Answer from the drawing. Dimensions are ordinates in mm from the lowest x, y and z of the part. Round coordinates to 2 decimals unless told otherwise and drop trailing zeros. Write each loop counter-clockwise with the first axis right and the second up, starting at its lowest first coordinate (ties: lowest second). Pieces come first, ordered by that corner, then holes. Notation, with made-up numbers: (-38, 32.5) -> (-1, 32.5) arc R21 cw to (-1, 56.5) -> close; hole circle Ø1 at (-27, 5). An arc over 180 degrees is marked (long way). Answer as a JSON object with one key per item and string values. Group by question number.
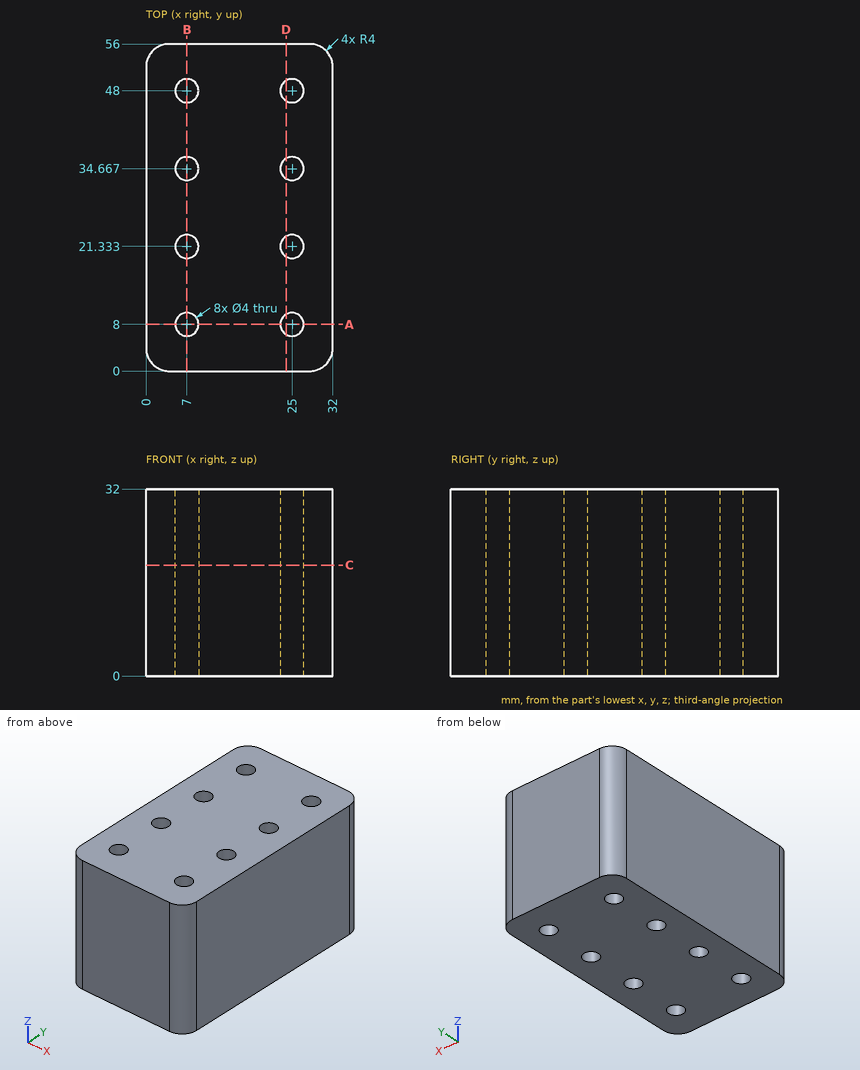
1) A cutting plane is placed at D-D on x = 24. Determine the outline of the cut face in (y, z) (1 decimal), plus the area to 3 significant figures.
2) Straight lines are drawn through the part: L1, parallel to Y at x = 25, z = 9.5; L2, parallel to X at y = 34.5, z = 14.5; L3, parallel to Y at x = 8.5, z = 15 (1 decimal). For each, find the intervals that lie inside material, in ascending order.
3) This flat-tipped pin is pushed along its axis until it touches: P1, Ø10, axis at x = 4.5, z = 7, coming from the -Y side. Where does it stop, or does it pass through?
4) A cutting plane is placed at A-A on y = 8. Determine the outline of the cut face in (x, z).
5) A cutting plane is placed at C-C on z = 19. State how many separate pieces and enclosed holes the cut face has, plus the area to 3 significant figures.
6) A cutting plane is placed at B-B on x = 7. Determine the outline of the cut face in (y, z).
Established:
{
 "1": {"outline": "(0, 0) -> (6.3, 0) -> (6.3, 32) -> (0, 32) -> close; (9.7, 0) -> (19.6, 0) -> (19.6, 32) -> (9.7, 32) -> close; (23.1, 0) -> (32.9, 0) -> (32.9, 32) -> (23.1, 32) -> close; (36.4, 0) -> (46.3, 0) -> (46.3, 32) -> (36.4, 32) -> close; (49.7, 0) -> (56, 0) -> (56, 32) -> (49.7, 32) -> close", "area": "1,350 mm²"},
 "2": {"L1": "y = 0 to 6, 10 to 19.33, 23.33 to 32.67, 36.67 to 46, 50 to 56", "L2": "x = 0 to 5.01, 8.99 to 23.01, 26.99 to 32", "L3": "y = 0 to 6.7, 9.3 to 20, 22.7 to 33.3, 36 to 46.7, 49.3 to 56"},
 "3": {"P1": "stops at y = 0"},
 "4": {"outline": "(0, 0) -> (5, 0) -> (5, 32) -> (0, 32) -> close; (9, 0) -> (23, 0) -> (23, 32) -> (9, 32) -> close; (27, 0) -> (32, 0) -> (32, 32) -> (27, 32) -> close"},
 "5": {"separate pieces": "1", "enclosed holes": "8", "area": "1,680 mm²"},
 "6": {"outline": "(0, 0) -> (6, 0) -> (6, 32) -> (0, 32) -> close; (10, 0) -> (19.33, 0) -> (19.33, 32) -> (10, 32) -> close; (23.33, 0) -> (32.67, 0) -> (32.67, 32) -> (23.33, 32) -> close; (36.67, 0) -> (46, 0) -> (46, 32) -> (36.67, 32) -> close; (50, 0) -> (56, 0) -> (56, 32) -> (50, 32) -> close"}
}
